For this review, take the finished solid that the model builds, in its own axes (mm). A direction names the side the tool comes from. Coordinates: 2 decimals unless noted, no trailing zeros. Write each loop counter-clockwise with the first axis right and the second up, starting at its lowest first coordinate (ties: lowest second). Pieces come first, ordered by that corner, then holes.
1) Insertion check: P1, Ø0.8, axis at x = 2.5, z = 39.5, coming from the -Y side; P2, Ø1.2, axis at x = 19.5, z = 51.5, coming from the +Y side. Each pin has a flat end and moves straight along its axis. Give the tip position at first contact, or say it passes through.
2) To check wall thickness, follow line 1 along X through (y, z) = (14, 88); line 2 along Y through (x, z) = (17.5, 89.5); line 3 along Y through (x, z) = (10, 73). State the ranges of each line that lie inside material, in increasing order.
3) We need section A-A on y = 10. Write out the cut boundary in (x, z).
4) For faces 1 (the face through (4, 0, 49)), 2 (the face through (5, 16, 49)), list the 3-axis set-ups (+Z, -Z, +X, -X, +Y, -Y) from which the entire face can be reached by the end or side of a thin tool; tool diameter is ignored.
5) Mouldability with a two-part tool opening along X and no side actions: class faces 3 (the face through (6, 1.5, 49)), 4 (the face through (0, 4, 49)), 5 (the face through (16, 20, 49)) as pulls with the +X half, pulls with the -X half, needs draft (parallel to the pull), parting line crosses it, or undercut.
from build123d import *

# Parameters (mm, degrees)
F0_R     = 3
F1_DEPTH = 100


with BuildPart() as f1:
    # F0 (on Top) → F1 (new body)
    with BuildSketch(Plane.XY):
        with BuildLine():
            ThreePointArc((0, 1.5), (0.43934, 0.43934), (1.5, 0))
            Line((1.5, 0), (7, 0))
            Line((7, 0), (7, 1.5))
            Line((7, 1.5), (4, 1.5))
            Line((4, 1.5), (4, 3))
            Line((4, 3), (6.5, 5.5))
            Line((6.5, 5.5), (10, 5.5))
            Line((10, 5.5), (13.5, 5.5))
            Line((13.5, 5.5), (16, 3))
            Line((16, 3), (16, 1.5))
            Line((16, 1.5), (13, 1.5))
            Line((13, 1.5), (13, 0))
            Line((13, 0), (18.5, 0))
            ThreePointArc((18.5, 0), (19.56066, 0.43934), (20, 1.5))
            Line((20, 1.5), (20, 7))
            Line((20, 7), (18.5, 7))
            Line((18.5, 7), (18.5, 4))
            Line((18.5, 4), (17, 4))
            Line((17, 4), (14.5, 6.5))
            Line((14.5, 6.5), (14.5, 10))
            Line((14.5, 10), (14.5, 13.5))
            Line((14.5, 13.5), (17, 16))
            Line((17, 16), (18.5, 16))
            Line((18.5, 16), (18.5, 13))
            Line((18.5, 13), (20, 13))
            Line((20, 13), (20, 18.5))
            ThreePointArc((20, 18.5), (19.56066, 19.56066), (18.5, 20))
            Line((18.5, 20), (13, 20))
            Line((13, 20), (13, 18.5))
            Line((13, 18.5), (16, 18.5))
            Line((16, 18.5), (16, 17))
            Line((16, 17), (13.5, 14.5))
            Line((13.5, 14.5), (10, 14.5))
            Line((10, 14.5), (6.5, 14.5))
            Line((6.5, 14.5), (4, 17))
            Line((4, 17), (4, 18.5))
            Line((4, 18.5), (7, 18.5))
            Line((7, 18.5), (7, 20))
            Line((7, 20), (1.5, 20))
            ThreePointArc((1.5, 20), (0.43934, 19.56066), (0, 18.5))
            Line((0, 18.5), (0, 13))
            Line((0, 13), (1.5, 13))
            Line((1.5, 13), (1.5, 16))
            Line((1.5, 16), (3, 16))
            Line((3, 16), (5.5, 13.5))
            Line((5.5, 13.5), (5.5, 10))
            Line((5.5, 10), (5.5, 6.5))
            Line((5.5, 6.5), (3, 4))
            Line((3, 4), (1.5, 4))
            Line((1.5, 4), (1.5, 7))
            Line((1.5, 7), (0, 7))
            Line((0, 7), (0, 1.5))
        make_face()
        with Locations((10, 10)):
            Circle(F0_R, mode=Mode.SUBTRACT)
    extrude(amount=F1_DEPTH)


solid = f1.part
Result:
1. P1: stops at y = 0
1. P2: stops at y = 19.95
2. line 1: x = 0 to 1.5, 5 to 15, 18.5 to 20
2. line 2: y = 0 to 4, 16 to 20
2. line 3: y = 5.5 to 7, 13 to 14.5
3. outline: (5.5, 0) - (7, 0) - (7, 100) - (5.5, 100) - close; (13, 0) - (14.5, 0) - (14.5, 100) - (13, 100) - close
4. face 1: +Z, -Z, +X, -X, -Y
4. face 2: +Z, -Z
5. face 3: undercut
5. face 4: pulls with the -X half
5. face 5: needs draft
